```python
from build123d import *

# Parameters (mm, degrees)
F0_W     = 20
F0_H     = 6
F1_DEPTH = 2
F2_T     = -2
F3_W     = 4
F3_H     = 2
F4_DEPTH = 25
F5_F1_R  = 0.9999
F5_F2_R  = 0.9999


# Not quite as in the source:
# - a fillet or chamfer is up to 0.001 mm smaller than in the source, because OpenCascade refuses the exact size


with BuildPart() as f1:
    # F0 (on Top) → F1 (new body)
    with BuildSketch(Plane.XY):
        with Locations((7.7290598062, 0.812693499)):
            Rectangle(F0_W, F0_H)
    extrude(amount=F1_DEPTH)

    # F2
    f2_openings = [f1.faces().sort_by_distance(p)[0] for p in [
        (7.72906, 0.812693, 2),
        (7.72906, 0.812693, 0),
    ]]
    offset(amount=F2_T, openings=f2_openings)

    # F3 (on face) → F4 (cut)
    with BuildSketch(Plane.XY.offset(2)):
        with Locations((7.7290598062, -1.187306501)):
            Rectangle(F3_W, F3_H)
    extrude(amount=-F4_DEPTH, mode=Mode.SUBTRACT)

    # F5: fillet of radius 1 on 8 edges, made by hand

    # F5_f1 (radius 1 in the source; OpenCascade refuses exactly that, so slightly less here)
    f5_f1_edges = [f1.edges().sort_by_distance(p)[0] for p in [
        (-0.2709401938, 1.812693499, 1),
        (-0.2709401938, -0.187306501, 1),
        (15.7290598062, -0.187306501, 1),
        (15.7290598062, 1.812693499, 1),
    ]]
    fillet(f5_f1_edges, radius=F5_F1_R)

    # F5_f2 (radius 1 in the source; OpenCascade refuses exactly that, so slightly less here)
    f5_f2_edges = [f1.edges().sort_by_distance(p)[0] for p in [
        (-0.2709401938, 0.812693499, 0),
        (-0.2709401938, 0.812693499, 2),
        (15.7290598062, 0.812693499, 0),
        (15.7290598062, 0.812693499, 2),
        (15.4361958767, 0.1055574285, 2),
        (15.4361958767, 1.5198295695, 2),
        (15.4361958767, 0.1055574285, 0),
        (15.4361958767, 1.5198295695, 0),
        (0.0219237357, 1.5198295695, 2),
        (0.0219237357, 0.1055574285, 2),
        (0.0219237357, 1.5198295695, 0),
        (0.0219237357, 0.1055574285, 0),
    ]]
    fillet(f5_f2_edges, radius=F5_F2_R)


solid = f1.part
```
Geometry: final body of the model. Coordinates: model frame, mm. A direction names the side the tool comes from. Coordinates: 2 decimals unless noted, no trailing zeros. Answer in a Markdown table with one row per item.
Item 1: Draft query along Y for faces 6 (the flat face through (9.729, -1, 1)), 7 (the cylindrical face through (3.194, -0.472, 1.699)), 8 (the flat face through (8, 3.813, 1)), 9 (the cylindrical face through (7.8, 2.1, 0.3)). Return one class per face: released by +Y, released by -Y, zero draft, split by the parting line, or undercut.
Return value:
| item | result |
|---|---|
| face 6 | zero draft |
| face 7 | undercut |
| face 8 | released by +Y |
| face 9 | undercut |
Item 2: Ray query, L1, parallel to X at y = -1.1, z = 1.6; L2, parallel to Y at x = 13, z = 1; L3, parallel to Z at x = 16.25, y = -0.4. Return the intervals inside material, ascending.
Return value:
| item | result |
|---|---|
| L1 | x = -2.27 to 5.73, 9.73 to 17.73 |
| L2 | y = -2.19 to -0.19, 1.81 to 3.81 |
| L3 | z = 0 to 2 |
Item 3: Access query for faces 1 (the flat face through (14, -2.187, 1)), 2 (the flat face through (5.729, -1, 1)), 3 (the cylindrical face through (3.194, -0.488, 0.285)), 4 (the flat face through (8, 3, 0)), 5 (the cylindrical face through (12.194, -0.472, 1.699)). Directions: +Z, -Z, +X, -X, +Y, -Y. A direction counts if a zero-diameter tool reaches every point of the face in a straight line with its end or side. Return the directions, or none.
Return value:
| item | result |
|---|---|
| face 1 | +Z, -Z, +X, -X, -Y |
| face 2 | +Z, -Z, -Y |
| face 3 | -Z |
| face 4 | -Z, +X, -X, +Y, -Y |
| face 5 | +Z |
